Geometry: final body of the model. Coordinates: model frame, mm. A direction names the side the tool comes from. Coordinates: 2 decimals unless noted, no trailing zeros. Order: outer loops, then holes, each group sorted by start corner. A loop starts at its lowest first (then second) coordinate and runs counter-clockwise, first axis right, second up. Notation, with made-up numbers: (-3.75, 64.25) -> (27.25, 64.25) arc R24 cw to (27.25, 87.25) -> close; hole circle Ø9 at (84, 40). An arc over 180 degrees is marked (long way). Use one line per item in the form item = value.
```python
from build123d import *

# Parameters (mm, degrees)
SKETCH1_W           = 68.747968374
SKETCH1_H           = 23.971240905
BOSS_EXTRUDE1_DEPTH = 9
SKETCH2_R           = 4
CUT_EXTRUDE1_DEPTH  = 9
FILLET1_R           = 2
SKETCH3_R           = 1.15
CUT_EXTRUDE2_DEPTH  = 5
CUT_EXTRUDE3_REACH  = 11
SKETCH4_R           = 4


with BuildPart() as part:
    # Sketch1 → Boss-Extrude1 (new body)
    with BuildSketch(Plane.ZY.offset(-74.969208633)):
        with Locations((20.319218255, 7.785620453)):
            Rectangle(SKETCH1_W, SKETCH1_H)
    extrude(amount=BOSS_EXTRUDE1_DEPTH)

    # Sketch2 → Cut-Extrude1 (cut)
    with BuildSketch(Plane.ZY.offset(-65.969208633)):
        with Locations((28, 7.3)):
            Circle(SKETCH2_R)
    extrude(amount=-CUT_EXTRUDE1_DEPTH, mode=Mode.SUBTRACT)

    # Fillet1
    fillet1_edges = [part.edges().sort_by_distance(p)[0] for p in [
        (70.469208633, 19.771240905, -14.054765932),
        (70.469208633, 19.771240905, 54.693202442),
        (70.469208633, -4.2, 54.693202442),
        (70.469208633, -4.2, -14.054765932),
    ]]
    fillet(fillet1_edges, radius=FILLET1_R)

    # Sketch3 → Cut-Extrude2 (cut)
    with BuildSketch(Plane(origin=(0, 19.771240905, 0), x_dir=(1, 0, 0), z_dir=(0, 1, 0))):
        with Locations((70.469208633, -42.659277992)):
            Circle(SKETCH3_R)
    extrude(amount=-CUT_EXTRUDE2_DEPTH, mode=Mode.SUBTRACT)

    # Sketch4 → Cut-Extrude3 (cut, up to next)
    with BuildSketch(Plane.ZY.offset(-65.969208633), mode=Mode.PRIVATE) as cut_extrude3_sk1:
        with Locations((-5.344766421, 7.785620452)):
            Circle(SKETCH4_R)
    cut_extrude3_tool1 = extrude(cut_extrude3_sk1.sketch, amount=-CUT_EXTRUDE3_REACH, mode=Mode.PRIVATE) & part.part
    add(cut_extrude3_tool1.solids().sort_by_distance((65.969209, 7.78562, -5.344766))[0], mode=Mode.SUBTRACT)


solid = part.part
```
1) Section B-B, the plane y = 8.75. Output: boundary loops of the cut face in (x, z).
Results found:
outline = (65.97, -14.05) -> (74.97, -14.05) -> (74.97, -9.23) -> (65.97, -9.23) -> close; (65.97, -1.46) -> (74.97, -1.46) -> (74.97, 24.27) -> (65.97, 24.27) -> close; (65.97, 31.73) -> (74.97, 31.73) -> (74.97, 54.69) -> (65.97, 54.69) -> close
2) Section C-C, the plane x = 67. Output: boundary loops of the cut face in (y, z), and give its area (3 significant figures).
Results found:
outline = (-4.2, -12.05) arc R2 ccw to (-2.2, -14.05) -> (17.77, -14.05) arc R2 ccw to (19.77, -12.05) -> (19.77, 52.69) arc R2 ccw to (17.77, 54.69) -> (-2.2, 54.69) arc R2 ccw to (-4.2, 52.69) -> close; hole circle Ø8 at (7.3, 28); hole circle Ø8 at (7.79, -5.34)
area = 1,540 mm2
3) Material intervals for probe 1 along Z at (x, y) = (71, 10); probe 2 along Z at (x, y) = (69.75, 7.25); probe 3 along Z at (x, y) = (70.5, 15.5), sorted ascending. Write a range as from..to.
Results found:
probe_1 = -14.05..-8.68, -2.01..25.05, 30.95..54.69
probe_2 = -14.05..-9.31, -1.38..24, 32..54.69
probe_3 = -14.05..41.51, 43.81..54.69
4) Section A-A, the plane z = 28. Output: boundary loops of the cut face in (x, y).
Results found:
outline = (65.97, -4.2) -> (74.97, -4.2) -> (74.97, 3.3) -> (65.97, 3.3) -> close; (65.97, 11.3) -> (74.97, 11.3) -> (74.97, 19.77) -> (65.97, 19.77) -> close
5) Pull-direction query (Y, two-part tool) for faces 3 (the flat face through (71, 19.771, 20)), 4 (the cylindrical face through (70.406, -3.599, -13.484)), 5 (the cylindrical face through (70.406, 7.476, 24.004)); classes: released by +Y, released by -Y, zero draft, split by the parting line, or undercut.
Results found:
face_3 = released by +Y
face_4 = released by -Y
face_5 = undercut
6) Access query for faces 1 (the cylindrical face through (70.41, 3.88, -6.21)), 2 (the cylindrical face through (69.557, 17.306, 43.359)). Directions: +Z, -Z, +X, -X, +Y, -Y. A direction counts if a zero-diameter tool reaches every point of the face in a straight line with its end or side. Return the directions, or none.
Results found:
face_1 = +X, -X
face_2 = +Y
